Design review of the part shown in the three views and the two pictorial views. Dimensions are in mm from the part's minimum x, y and z. A direction names the side the tool comes from. Round coordinates to 2 decimals unless told otherwise and drop trailing zeros. Loops run counter-clockwise (first coordinate to the right, second up) from the corner with the lowest first, then second, coordinate; pieces in that order, holes last. Notation, with made-up numbers: M 3.5,81 L 12.5,81 A6 ccw 12.5,88 Z; hole C -28.75,74.25 d3. An arc over 180 degrees is marked long. Return JSON: item names as keys, results as strings. Group by question number.
Q1. Consider section D-D (x = 66). State the section outline as (y, z) points (3 decimals), and give its area (3 significant figures).
Q2. To check wall thickness, follow line 1 along Y through (x, z) = (44, 4.95); line 2 along Y through (x, z) = (34, 3.75); line 3 along X through (y, z) = (28, 3.55). State the ranges of each line that lie inside material, in increasing order.
Q3. Consider section A-A (y = 49). State the section outline as (x, z) points (3 decimals), and give its area (3 significant figures).
Q4. Consider section B-B (z = 2). State the section outline as (x, y) points.
Q5. Clearance check with flat-ended pins moving along their axes: pin 1 Ø2 at (y, z) = (24, 2.5) entering from +X; pin 2 Ø3 at (x, z) = (65, 4) entering from +Y; pin 3 Ø3 at (y, z) = (46, 3) entering from -X; pin 4 Ø3 at (y, z) = (60.5, 2.5) entering from -X. State where each tip first meets the part, or that it passes through.
Q6. For the marked faces 1, 2, 3 and 4, list the 3-axis set-ups (+Z, -Z, +X, -X, +Y, -Y) from which the entire face can be reached by the end or side of a thin tool; tool diameter is ignored.
Q7. Draft analysis for pull direction X (two halves, no side actions). For the marked faces 5, 6, 7 and 8, state which applies: pulls with the +X half, pulls with the -X half, needs draft (parallel to the pull), parting line crosses it, or undercut.
Q8. Consider section C-C (y = 31). State the section outline as (x, z) points (1 decimal).
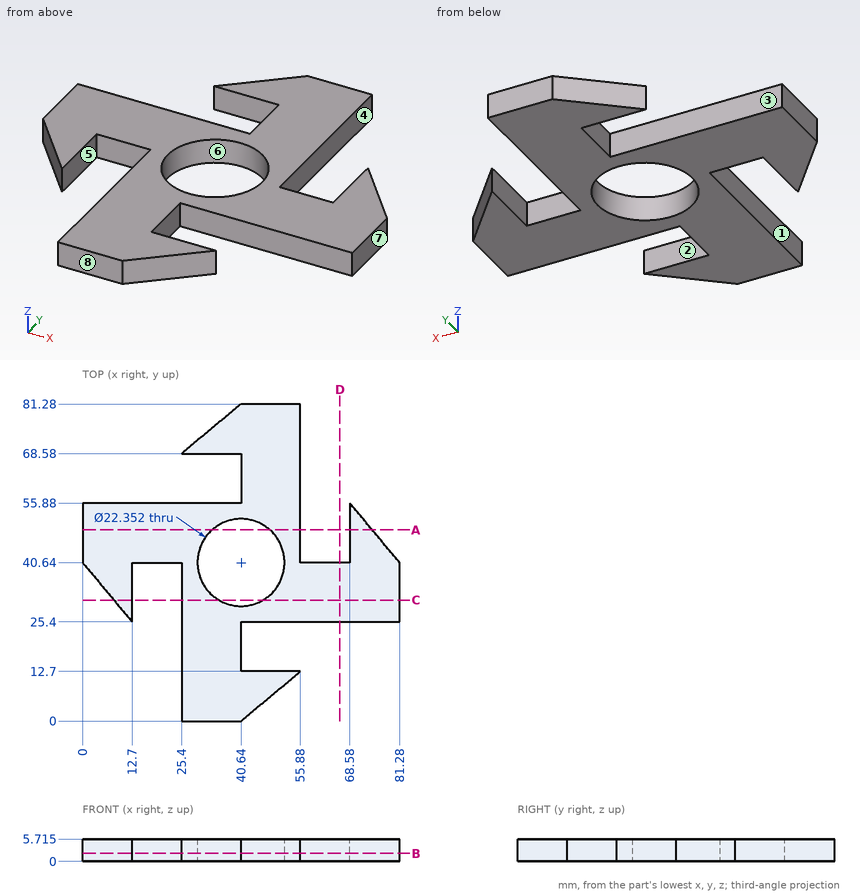
Values:
{
 "1": {"outline": "M 25.4,0 L 40.64,0 L 40.64,5.715 L 25.4,5.715 Z", "area": "87.1 mm2"},
 "2": {"line 1": "y = 2.8 to 12.7, 25.4 to 29.98, 51.3 to 81.28", "line 2": "y = 0 to 31.65, 49.63 to 55.88, 68.58 to 75.75", "line 3": "x = 10.53 to 12.7, 25.4 to 81.28"},
 "3": {"outline": "M 0,0 L 33.223,0 L 33.223,5.715 L 0,5.715 Z; M 48.057,0 L 55.88,0 L 55.88,5.715 L 48.057,5.715 Z; M 68.58,0 L 74.313,0 L 74.313,5.715 L 68.58,5.715 Z", "area": "267 mm2"},
 "4": {"outline": "M 0,40.64 L 12.7,25.4 L 12.7,40.64 L 25.4,40.64 L 25.4,0 L 40.64,0 L 55.88,12.7 L 40.64,12.7 L 40.64,25.4 L 81.28,25.4 L 81.28,40.64 L 68.58,55.88 L 68.58,40.64 L 55.88,40.64 L 55.88,81.28 L 40.64,81.28 L 25.4,68.58 L 40.64,68.58 L 40.64,55.88 L 0,55.88 Z; hole C 40.64,40.64 d22.35"},
 "5": {"pin 1": "stops at x = 40.64", "pin 2": "stops at y = 40.64", "pin 3": "stops at x = 0", "pin 4": "stops at x = 40.64"},
 "6": {"face 1": "+Z, -Z, -Y", "face 2": "+Z, -Z, +X", "face 3": "+Z, -Z, -X", "face 4": "+Z, -Z, +Y"},
 "7": {"face 5": "undercut", "face 6": "undercut", "face 7": "pulls with the +X half", "face 8": "needs draft"},
 "8": {"outline": "M 8,0 L 12.7,0 L 12.7,5.7 L 8,5.7 Z; M 25.4,0 L 35,0 L 35,5.7 L 25.4,5.7 Z; M 46.3,0 L 81.3,0 L 81.3,5.7 L 46.3,5.7 Z"}
}
